from build123d import *

# Parameters (mm, degrees)
BOSS_EXTRUDE1_DEPTH = 2
CUT_EXTRUDE2_DEPTH  = 1


with BuildPart() as part:
    # Sketch3 → Boss-Extrude1 (new body)
    with BuildSketch(Plane.XY):
        Polygon((146.625606574, 159.719339874), (183.625606574, 159.719339874), (185.625606574, 157.719339874), (185.625606574, 136.719339874), (183.625606574, 134.719339874), (146.625606574, 134.719339874), (144.625606574, 136.719339874), (144.625606574, 157.719339874), align=None)
    extrude(amount=BOSS_EXTRUDE1_DEPTH)

    # Sketch4 → Cut-Extrude2 (cut)
    with BuildSketch(Plane.XY):
        with BuildLine():
            Line((183.985590549, 149.719355145), (183.985590549, 144.719355145))
            ThreePointArc((183.985590549, 144.719355145), (182.485590549, 143.219355145), (180.985590549, 144.719355145))
            Line((180.985590549, 144.719355145), (180.985590549, 146.219355145))
            Line((180.985590549, 146.219355145), (172.842061199, 146.219355145))
            Line((172.842061199, 146.219355145), (168.466892344, 142.221525657))
            ThreePointArc((168.466892344, 142.221525657), (164.985590549, 140.717307295), (161.504288754, 142.221525657))
            Line((161.504288754, 142.221525657), (156.8366409, 146.486989717))
            ThreePointArc((156.8366409, 146.486989717), (156.485875357, 147.242486304), (156.873407646, 147.979799185))
            Line((156.873407646, 147.979799185), (161.520046065, 152.231799364))
            ThreePointArc((161.520046065, 152.231799364), (164.985590549, 153.719355145), (168.451135032, 152.231799364))
            Line((168.451135032, 152.231799364), (172.836292086, 148.219355145))
            Line((172.836292086, 148.219355145), (180.985590549, 148.219355145))
            Line((180.985590549, 148.219355145), (180.985590549, 149.719355145))
            ThreePointArc((180.985590549, 149.719355145), (182.485590549, 151.219355145), (183.985590549, 149.719355145))
        make_face()
    extrude(amount=CUT_EXTRUDE2_DEPTH, mode=Mode.SUBTRACT)


solid = part.part
Geometry: final body of the model. Coordinates: model frame, mm. A direction names the side the tool comes from. Give positions to 0.01 mm unless a question says otherwise; leave off trailing zeros. Order: outer loops, then holes, each group sorted by start corner. A loop starts at its lowest first (then second) coordinate and runs counter-clockwise, first axis right, second up. Notation, with made-up numbers: (40.5, -30.75) -> (58.5, -30.75) arc R27 cw to (58.5, -13.75) -> close; hole circle Ø5 at (42, -35.5). An arc over 180 degrees is marked (long way). Answer as a JSON object with one key per item and string values.
Q1. Section C-C (y = 143.75). Output: boundary loops of the cut face in (x, z), plus the area to 3 significant figures.
Entries:
{"outline": "(144.63, 0) -> (159.83, 0) -> (159.83, 1) -> (170.14, 1) -> (170.14, 0) -> (181.34, 0) -> (181.34, 1) -> (183.63, 1) -> (183.63, 0) -> (185.63, 0) -> (185.63, 2) -> (144.63, 2) -> close", "area": "69.4 mm^2"}
Q2. Access query for faces 4 (the flat face through (180.986, 145.5, 0.5)), 5 (the flat face through (165, 134.719, 1)). Directions: +Z, -Z, +X, -X, +Y, -Y. A direction counts if a zero-diameter tool reaches every point of the face in a straight line with its end or side. Return the directions, or none.
Entries:
{"face 4": "-Z", "face 5": "+Z, -Z, +X, -X, -Y"}
Q3. Material intervals for probe 1 along X at (y, z) = (150.25, 0.8); probe 2 along X at (y, z) = (150, 0.5); probe 3 along X at (y, z) = (147.5, 0.9), sorted ascending.
Entries:
{"probe 1": "x = 144.63 to 159.35, 170.62 to 181.08, 183.89 to 185.63", "probe 2": "x = 144.63 to 159.08, 170.89 to 181.01, 183.96 to 185.63", "probe 3": "x = 144.63 to 156.53, 183.99 to 185.63"}
Q4. Section B-B (x = 166.5). Output: boundary loops of the cut face in (y, z).
Entries:
{"outline": "(134.72, 0) -> (140.96, 0) -> (140.96, 1) -> (153.47, 1) -> (153.47, 0) -> (159.72, 0) -> (159.72, 2) -> (134.72, 2) -> close"}
Q5. Section D-D (x = 172). Output: boundary loops of the cut face in (y, z).
Entries:
{"outline": "(134.72, 0) -> (145.45, 0) -> (145.45, 1) -> (148.98, 1) -> (148.98, 0) -> (159.72, 0) -> (159.72, 2) -> (134.72, 2) -> close"}
Q6. Section A-A (z = 0.7). Output: boundary loops of the cut face in (x, y), plus the area to 3 significant figures.
Entries:
{"outline": "(144.63, 136.72) -> (146.63, 134.72) -> (183.63, 134.72) -> (185.63, 136.72) -> (185.63, 157.72) -> (183.63, 159.72) -> (146.63, 159.72) -> (144.63, 157.72) -> close; hole (156.84, 146.49) -> (161.5, 142.22) arc R4.78 ccw to (168.47, 142.22) -> (172.84, 146.22) -> (180.99, 146.22) -> (180.99, 144.72) arc R1.5 ccw to (183.99, 144.72) -> (183.99, 149.72) arc R1.5 ccw to (180.99, 149.72) -> (180.99, 148.22) -> (172.84, 148.22) -> (168.45, 152.23) arc R4.78 ccw to (161.52, 152.23) -> (156.87, 147.98) arc R0.94 ccw to start", "area": "841 mm^2"}
Q7. Draft query along Y for faces 1 (the flat face through (165, 159.719, 1)), 2 (the flat face through (144.626, 147, 1)), 3 (the flat face through (170.685, 144.248, 0.493)). Return one class per face: released by +Y, released by -Y, zero draft, split by the parting line, or undercut.
Entries:
{"face 1": "released by +Y", "face 2": "zero draft", "face 3": "undercut"}
Q8. First-contact query: pin 1 (2 mm diameter, centred on x = 167, y = 152.5, fed in from -Z). Flat tip, straight axial feed; report the tip coordinate or a pass-through.
Entries:
{"pin 1": "stops at z = 0"}
